Geometry check sheet. Reference: drawing and pictorial views, mm from the part's lowest x, y, z. Round coordinates to 2 decimals unless told otherwise and drop trailing zeros. Write each loop counter-clockwise with the first axis right and the second up, starting at its lowest first coordinate (ties: lowest second). Pieces come first, ordered by that corner, then holes. Notation, with made-up numbers: M -24.5,43.25 L 7.5,43.25 A14 ccw 7.5,50.25 Z; hole C -37.75,38.25 d7. An arc over 180 degrees is marked long. One line per question, with ' | ' between items.
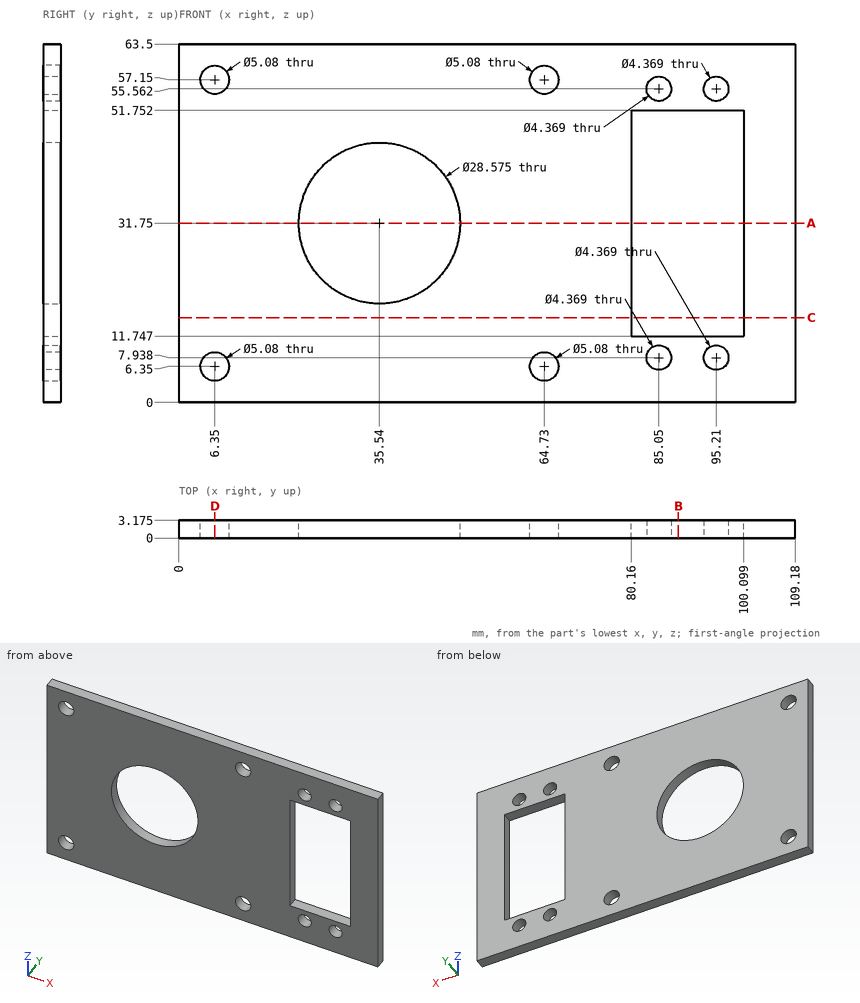
1. Section check D-D, the plane x = 6.35. Record the cut outline in (y, z) (1 decimal).
Results:
outline: M 0,0 L 3.2,0 L 3.2,3.8 L 0,3.8 Z; M 0,8.9 L 3.2,8.9 L 3.2,54.6 L 0,54.6 Z; M 0,59.7 L 3.2,59.7 L 3.2,63.5 L 0,63.5 Z
2. Section check C-C, the plane z = 15. Record the cut outline in (x, y) (1 decimal).
Results:
outline: M 0,0 L 80.2,0 L 80.2,3.2 L 0,3.2 Z; M 100.1,0 L 109.2,0 L 109.2,3.2 L 100.1,3.2 Z
3. Section check B-B, the plane x = 88.5. Record the cut outline in (y, z) (1 decimal).
Results:
outline: M 0,0 L 3.2,0 L 3.2,11.7 L 0,11.7 Z; M 0,51.8 L 3.2,51.8 L 3.2,63.5 L 0,63.5 Z
4. Thickness scan on line 1 (X direction, y = 1.2, z = 31.75); line 2 (Z direction, x = 6.35, y = 2.5); line 3 (Z direction, x = 87.5, y = 0.9). Record the ranges inside material, lowest first.
Results:
line 1: x = 0 to 21.25, 49.83 to 80.16, 100.1 to 109.18 | line 2: z = 0 to 3.81, 8.89 to 54.61, 59.69 to 63.5 | line 3: z = 0 to 11.75, 51.75 to 63.5
5. Section check A-A, the plane z = 31.75. Record the cut outline in (x, y) (1 decimal).
Results:
outline: M 0,0 L 21.3,0 L 21.3,3.2 L 0,3.2 Z; M 49.8,0 L 80.2,0 L 80.2,3.2 L 49.8,3.2 Z; M 100.1,0 L 109.2,0 L 109.2,3.2 L 100.1,3.2 Z
6. Go/stop test with a flat-tipped pin: P1, Ø4, axis at x = 95.21, z = 7.94, coming from the +Y side. Record where the tip stops, or that it passes through.
Results:
P1: passes through
